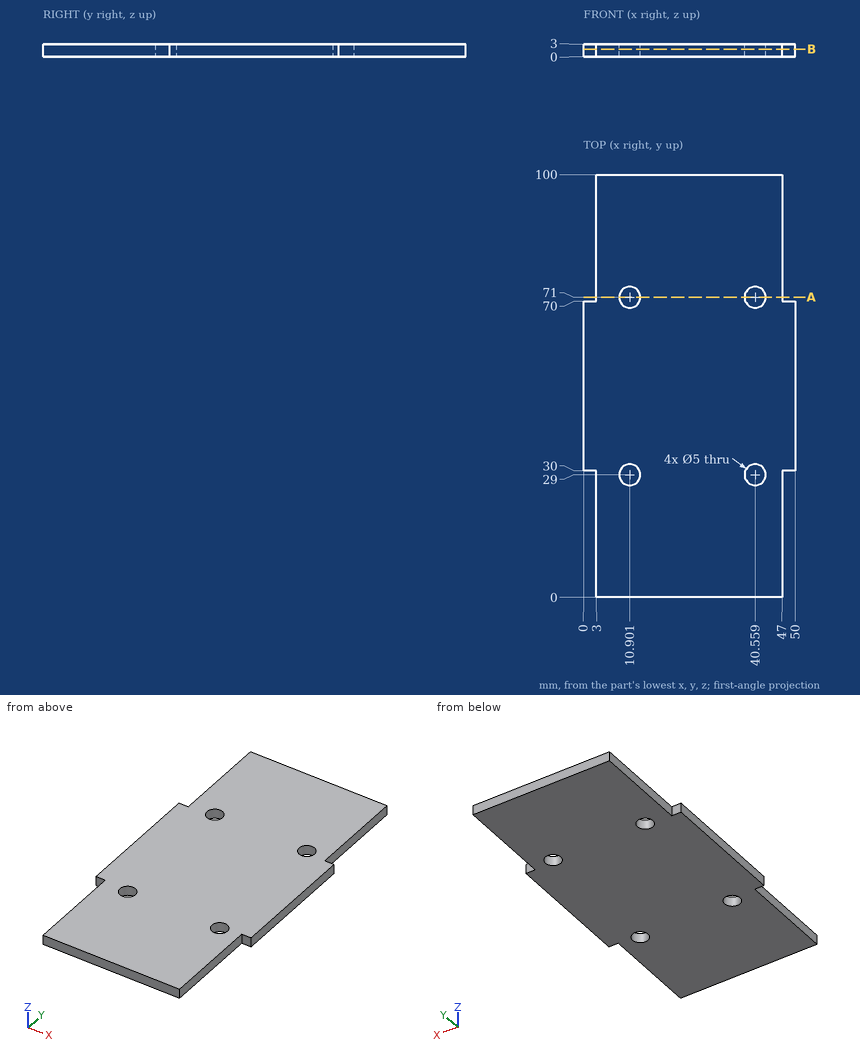
Geometry check sheet. Reference: drawing and pictorial views, mm from the part's lowest x, y, z. Give positions to 0.01 mm unless a question says otherwise; leave off trailing zeros. Write each loop counter-clockwise with the first axis right and the second up, starting at its lowest first coordinate (ties: lowest second). Pieces come first, ordered by that corner, then holes. Notation, with made-up numbers: (31, 70) -> (67, 70) arc R31 cw to (67, 96) -> close; hole circle Ø6 at (53, 86.25). An arc over 180 degrees is marked (long way). One line per item, written item: value. Start each with the question number.
Item 1: Section check B-B on z = 1.8. Record the cut outline in (x, y).
Item 2: Section check A-A on y = 71. Record the cut outline in (x, z).
Item 3: Gauge pin test, flat ends, axial feed: pin 1 (1.5 mm diameter, centred on y = 19.5, z = 1, fed in from +X); pin 2 (1.5 mm diameter, centred on x = 48.5, z = 2, fed in from -Y); pin 3 (1.5 mm diameter, centred on x = 49, z = 1, fed in from +Y); pin 4 (4.5 mm diameter, centred on x = 40.56, y = 29, fed in from -Z). Record the tip position at first contact, or that the pin passes through.
Item 4: Material ranges on probe 1 along Y at (x, z) = (11, 2.45); probe 2 along X at (y, z) = (29, 1.7); probe 3 along Y at (x, z) = (10, 2.7), recorded low to high. Write a range as from..to.
Results list:
1. outline: (0, 30) -> (3, 30) -> (3, 0) -> (47, 0) -> (47, 30) -> (50, 30) -> (50, 70) -> (47, 70) -> (47, 100) -> (3, 100) -> (3, 70) -> (0, 70) -> close; hole circle Ø5 at (10.9, 29); hole circle Ø5 at (10.9, 71); hole circle Ø5 at (40.56, 29); hole circle Ø5 at (40.56, 71)
2. outline: (3, 0) -> (8.4, 0) -> (8.4, 3) -> (3, 3) -> close; (13.4, 0) -> (38.06, 0) -> (38.06, 3) -> (13.4, 3) -> close; (43.06, 0) -> (47, 0) -> (47, 3) -> (43.06, 3) -> close
3. pin 1: x = 47
3. pin 2: y = 30
3. pin 3: y = 70
3. pin 4: through
4. probe 1: 0..26.5, 31.5..68.5, 73.5..100
4. probe 2: 3..8.4, 13.4..38.06, 43.06..47
4. probe 3: 0..26.67, 31.33..68.67, 73.33..100
